Print and shaded views of the part. All mm, measured from the part's lowest x, y and z. Round coordinates to 2 decimals unless told otherwise and drop trailing zeros. Write each loop counter-clockwise with the first axis right and the second up, starting at its lowest first coordinate (ties: lowest second). Pieces come first, ordered by that corner, then holes. Notation, with made-up numbers: M 62.5,-1.5 L 100.5,-1.5 A25 ccw 100.5,36.5 Z; hole C -25,31.25 d11. An arc over 180 degrees is marked long. Write item = value, one per line.
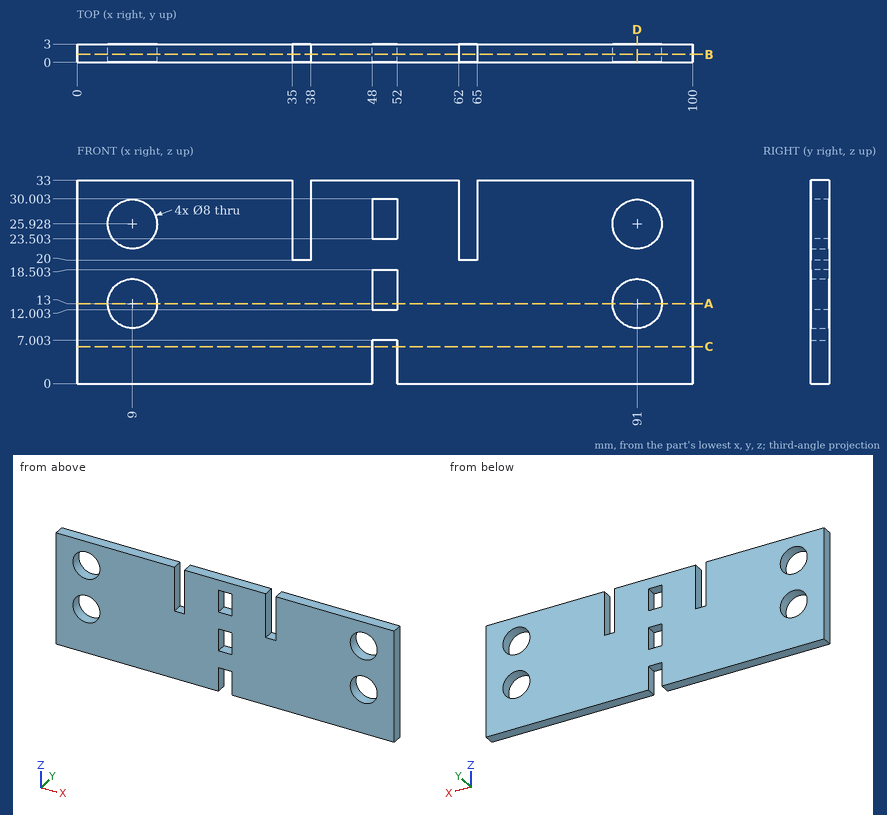
1. Band-saw the part on D-D (x = 91). List the corners of the cut face in (y, z).
Responses:
outline = M 0,0 L 3,0 L 3,9 L 0,9 Z; M 0,17 L 3,17 L 3,21.93 L 0,21.93 Z; M 0,29.93 L 3,29.93 L 3,33 L 0,33 Z
2. Band-saw the part on C-C (z = 6). List the corners of the cut face in (x, y), plus the area to 3 significant figures.
Responses:
outline = M 0,0 L 48,0 L 48,3 L 0,3 Z; M 52,0 L 100,0 L 100,3 L 52,3 Z
area = 288 mm²
3. Band-saw the part on B-B (y = 1.3). List the corners of the cut face in (x, z).
Responses:
outline = M 0,0 L 48,0 L 48,7 L 52,7 L 52,0 L 100,0 L 100,33 L 65,33 L 65,20 L 62,20 L 62,33 L 38,33 L 38,20 L 35,20 L 35,33 L 0,33 Z; hole C 9,13 d8; hole C 9,25.93 d8; hole M 48,12 L 52,12 L 52,18.5 L 48,18.5 Z; hole M 48,23.5 L 52,23.5 L 52,30 L 48,30 Z; hole C 91,13 d8; hole C 91,25.93 d8
4. Flat gauge pins, fed straight in: pin 1 (0.9 mm diameter, centred on x = 37, y = 1, fed in from +Z); pin 2 (1.5 mm diameter, centred on x = 50, y = 1, fed in from -Z). Where does each tip first touch, or does it go through?
Responses:
pin_1 = 20
pin_2 = 7
5. Band-saw the part on A-A (z = 13). List the corners of the cut face in (x, y), plus the area to 3 significant figures.
Responses:
outline = M 0,0 L 5,0 L 5,3 L 0,3 Z; M 13,0 L 48,0 L 48,3 L 13,3 Z; M 52,0 L 87,0 L 87,3 L 52,3 Z; M 95,0 L 100,0 L 100,3 L 95,3 Z
area = 240 mm²
6. Probe probe 1 along X at (y, z) = (1.2, 21.5); probe 2 along Z at (x, y) = (51.5, 1); probe 3 along X at (y, z) = (1.5, 13). List the from-to ranges inside material, lowest first.
Responses:
probe_1 = 0 to 35, 38 to 62, 65 to 100
probe_2 = 7 to 12, 18.5 to 23.5, 30 to 33
probe_3 = 0 to 5, 13 to 48, 52 to 87, 95 to 100
